Source: CAD feature listing. Evaluate the final solid. Frame: model axes, mm. A direction names the side the tool comes from. Round coordinates to 2 decimals unless told otherwise and drop trailing zeros. Order: outer loops, then holes, each group sorted by start corner. A loop starts at its lowest first (then second) coordinate and runs counter-clockwise, first axis right, second up. Notation, with made-up numbers: (-1.5, 29) -> (22.5, 29) arc R13 cw to (22.5, 38) -> close; hole circle Ø10 at (34, 43.25). An arc over 180 degrees is marked (long way). Use a Markdown table: item, result. Add a question column.
```python
from build123d import *

# Parameters (mm, degrees)
SKETCH1_R               = 6
BOSS_EXTRUDE1_DEPTH     = 20
SKETCH2_R               = 3.4
CUT_EXTRUDE1_DEPTH      = 13.55
SKETCH5_W               = 1.550685087
SKETCH5_H               = 7.184215806
BOSS_EXTRUDE2_DEPTH     = 13.55
SKETCH7_W               = 18.003976239
SKETCH7_H               = 19.909960041
BOSS_EXTRUDE3_DEPTH     = 10
SKETCH6_R               = 2
CUT_EXTRUDE2_DEPTH      = 1
CUT_EXTRUDE2_DEPTH_BACK = 13.55
CUT_EXTRUDE3_DEPTH      = 10
CUT_EXTRUDE3_DEPTH_BACK = 10
SKETCH10_R              = 50
BOSS_EXTRUDE4_DEPTH     = 30
SKETCH11_R              = 5
CUT_EXTRUDE4_DEPTH      = 30
SKETCH12_R              = 42.124366513
SKETCH12_R_2            = 15.95790089
CUT_EXTRUDE5_DEPTH      = 27


with BuildPart() as part:
    # Sketch1 → Boss-Extrude1 (new body)
    with BuildSketch(Plane(origin=(0, 0, 0), x_dir=(1, 0, 0), z_dir=(0, 1, 0))):
        Circle(SKETCH1_R)
    extrude(amount=BOSS_EXTRUDE1_DEPTH)

    # Sketch2 → Cut-Extrude1 (cut)
    with BuildSketch(Plane(origin=(0, 20, 0), x_dir=(1, 0, 0), z_dir=(0, 1, 0))):
        Circle(SKETCH2_R)
    extrude(amount=-CUT_EXTRUDE1_DEPTH, mode=Mode.SUBTRACT)

    # Sketch5 → Boss-Extrude2 (add)
    with BuildSketch(Plane(origin=(0, 18.26, 0), x_dir=(1, 0, 0), z_dir=(0, 1, 0))):
        with Locations((3.375342544, 0.020519704)):
            Rectangle(SKETCH5_W, SKETCH5_H)
    extrude(amount=-BOSS_EXTRUDE2_DEPTH)

    # Sketch7 → Boss-Extrude3 (add)
    with BuildSketch(Plane.ZY.offset(-2.6)):
        with Locations((0.33027221, 9.954980021)):
            Rectangle(SKETCH7_W, SKETCH7_H)
    extrude(amount=-BOSS_EXTRUDE3_DEPTH)

    # Sketch6 → Cut-Extrude2 (cut, two sides)
    with BuildSketch(Plane.ZY.offset(-2.6)) as cut_extrude2_sk:
        with Locations((0, 10.236925537)):
            Circle(SKETCH6_R)
    extrude(amount=CUT_EXTRUDE2_DEPTH, mode=Mode.SUBTRACT)
    extrude(cut_extrude2_sk.sketch, amount=-CUT_EXTRUDE2_DEPTH_BACK, mode=Mode.SUBTRACT)

    # Sketch9 → Cut-Extrude3 (cut, two sides)
    with BuildSketch(Plane.XY) as cut_extrude3_sk:
        Polygon((10.876516382, 10.236925537), (10.876516382, 5.861925537), (4.943430227, 5.861925537), (4.943430227, 10.236925537), (4.943430227, 14.614332445), (10.876516382, 14.614332445), align=None)
    extrude(amount=CUT_EXTRUDE3_DEPTH, mode=Mode.SUBTRACT)
    extrude(cut_extrude3_sk.sketch, amount=-CUT_EXTRUDE3_DEPTH_BACK, mode=Mode.SUBTRACT)

    # Sketch10 → Boss-Extrude4 (add)
    with BuildSketch(Plane.XZ):
        Circle(SKETCH10_R)
    extrude(amount=BOSS_EXTRUDE4_DEPTH)

    # Sketch11 → Cut-Extrude4 (cut)
    with BuildSketch(Plane(origin=(0, 0, 0), x_dir=(1, 0, 0), z_dir=(0, 1, 0))):
        with Locations((5, -49.946157791)):
            Circle(SKETCH11_R)
        with Locations((-14.494169434, -48.057650072)):
            Circle(SKETCH11_R)
        with Locations((-31.781732962, -38.852800774)):
            Circle(SKETCH11_R)
        with Locations((-44.230815749, -23.732964759)):
            Circle(SKETCH11_R)
        with Locations((-49.946157791, -5)):
            Circle(SKETCH11_R)
        with Locations((-48.057650072, 14.494169434)):
            Circle(SKETCH11_R)
        with Locations((-38.852800774, 31.781732962)):
            Circle(SKETCH11_R)
        with Locations((-23.732964759, 44.230815749)):
            Circle(SKETCH11_R)
        with Locations((-5, 49.946157791)):
            Circle(SKETCH11_R)
        with Locations((14.494169434, 48.057650072)):
            Circle(SKETCH11_R)
        with Locations((31.781732962, 38.852800774)):
            Circle(SKETCH11_R)
        with Locations((44.230815749, 23.732964759)):
            Circle(SKETCH11_R)
        with Locations((49.946157791, 5)):
            Circle(SKETCH11_R)
        with Locations((48.057650072, -14.494169434)):
            Circle(SKETCH11_R)
        with Locations((38.852800774, -31.781732962)):
            Circle(SKETCH11_R)
        with Locations((23.732964759, -44.230815749)):
            Circle(SKETCH11_R)
    extrude(amount=-CUT_EXTRUDE4_DEPTH, mode=Mode.SUBTRACT)

    # Sketch12 → Cut-Extrude5 (cut)
    with BuildSketch(Plane(origin=(0, 0, 0), x_dir=(1, 0, 0), z_dir=(0, 1, 0))):
        Circle(SKETCH12_R)
        Circle(SKETCH12_R_2, mode=Mode.SUBTRACT)
    extrude(amount=-CUT_EXTRUDE5_DEPTH, mode=Mode.SUBTRACT)


solid = part.part
```
1) Section B-B on z = 12. Output: boundary loops of the cut face in (x, y), then the cut area to 3 significant figures.
2) First-contact query: pin 1 Ø8 at (x, z) = (7, 1.5) entering from +Y; pin 2 Ø1 at (x, z) = (-6, 25.5) entering from +Y; pin 3 Ø5 at (x, y) = (37.5, -4) entering from +Z; pin 4 Ø4.5 at (y, z) = (11, -2.5) entering from +X. Flat tips, straight axial feed; report the tip coordinate or a pass-through.
3) Reachability of faces 1 (the flat face through (10.877, 10.2, 2.5)), 2 (the cylindrical face through (15.22, -13.31, -4.79)), 3 (the cylindrical face through (4.754, -14.79, -49.773)), 4 (the flat face through (3, 20, 3)), 5 (the flat face through (4, 10, 9.332)) from +Z, -Z, +X, -X, +Y, -Y: full face, straight path, thin tool, end or side. Return the list, or none.
4) Draft query along Z for faces 6 (the flat face through (-34, 0, -26)), 7 (the cylindrical face through (44.165, -14.79, 23.44)), 8 (the cylindrical face through (11.73, 12.22, -0.26)), 9 (the cylindrical face through (3.76, 12.22, -0.26)). Return one class per face: pulls with the +Z half, pulls with the -Z half, needs draft (parallel to the pull), parting line crosses it, or undercut.
5) Section A-A on y = -18. Count the separate pieces of the cut face and the enclosed holes in it, then the cut area to 3 significant figures.
6) Line query: probe 1 along X at (y, z) = (14.25, 0); probe 2 along Y at (x, z) = (4.2, 0); probe 3 along X at (y, z) = (-24, -8). Output: solid intervals per line, ascending. Write a range as from..to.
Conclusion:
| question | item | result |
|---|---|---|
| 1 | outline | (-48.54, -30) -> (43.72, -30) -> (43.72, 0) -> (40.38, 0) -> (40.38, -27) -> (10.52, -27) -> (10.52, 0) -> (-10.52, 0) -> (-10.52, -27) -> (-40.38, -27) -> (-40.38, 0) -> (-48.54, 0) -> close |
| 1 | area | 1,160 mm^2 |
| 2 | pin 1 | stops at y = 20 |
| 2 | pin 2 | stops at y = -27 |
| 2 | pin 3 | stops at z = 35.71 |
| 2 | pin 4 | stops at x = 12.6 |
| 3 | face 1 | +Z, -Z |
| 3 | face 2 | +Y |
| 3 | face 3 | -Z, +X, +Y, -Y |
| 3 | face 4 | +Z, -Z, +X, -X, +Y |
| 3 | face 5 | +Z, +X, -X, +Y |
| 4 | face 6 | needs draft |
| 4 | face 7 | pulls with the +Z half |
| 4 | face 8 | undercut |
| 4 | face 9 | undercut |
| 5 | separate pieces | 2 |
| 5 | enclosed holes | 1 |
| 5 | area | 2,500 mm^2 |
| 6 | probe 1 | x = -6..-3.4, 2.6..4.94, 10.88..12.6 |
| 6 | probe 2 | y = -30..8.24, 12.24..20 |
| 6 | probe 3 | x = -49.36..-41.36, -13.81..13.81, 41.36..45.95 |
